```python
from build123d import *

# Parameters (mm, degrees)
SKETCH1_W                                         = 172.72
SKETCH1_H                                         = 64.77
BOSS_EXTRUDE1_DEPTH                               = 1.5875
CSK_FOR_8_FLAT_HEAD_MACHINE_SCREW_100_D           = 4.4958
CSK_FOR_8_FLAT_HEAD_MACHINE_SCREW_100_DEPTH       = 12.7
CSK_FOR_8_FLAT_HEAD_MACHINE_SCREW_100_CSINK_D     = 8.4328
CSK_FOR_8_FLAT_HEAD_MACHINE_SCREW_100_CSINK_ANGLE = 100
CSK_FOR_8_FLAT_HEAD_MACHINE_SCREW_100_TIP         = 1.350674586


with BuildPart() as part:
    # Sketch1 → Boss-Extrude1 (new body)
    with BuildSketch(Plane(origin=(0, 0, 0), x_dir=(1, 0, 0), z_dir=(0, 1, 0))):
        with Locations((86.36, 32.385)):
            Rectangle(SKETCH1_W, SKETCH1_H)
    extrude(amount=BOSS_EXTRUDE1_DEPTH)

    # CSK for #8 Flat Head Machine Screw (100)1
    with Locations(Plane(origin=(0, 1.5875, 0), x_dir=(1, 0, 0), z_dir=(0, 1, 0))):
        with Locations((12.7, 54.61), (38.1, 54.61), (63.5, 54.61), (109.22, 54.61), (134.62, 54.61), (160.02, 54.61), (160.02, 10.16), (134.62, 10.16), (109.22, 10.16), (63.5, 10.16), (38.1, 10.16), (12.7, 10.16)):
            CounterSinkHole(CSK_FOR_8_FLAT_HEAD_MACHINE_SCREW_100_D / 2, CSK_FOR_8_FLAT_HEAD_MACHINE_SCREW_100_CSINK_D / 2, depth=CSK_FOR_8_FLAT_HEAD_MACHINE_SCREW_100_DEPTH, counter_sink_angle=CSK_FOR_8_FLAT_HEAD_MACHINE_SCREW_100_CSINK_ANGLE)
            with Locations((0, 0, -(CSK_FOR_8_FLAT_HEAD_MACHINE_SCREW_100_DEPTH + CSK_FOR_8_FLAT_HEAD_MACHINE_SCREW_100_TIP / 2))):  # 118° drill point
                Cone(0, CSK_FOR_8_FLAT_HEAD_MACHINE_SCREW_100_D / 2, CSK_FOR_8_FLAT_HEAD_MACHINE_SCREW_100_TIP, mode=Mode.SUBTRACT)


solid = part.part
```
Geometry check sheet. Reference: the model listing, model coordinates, mm. Coordinates: 2 decimals unless noted, no trailing zeros. Order: outer loops, then holes, each group sorted by start corner. A loop starts at its lowest first (then second) coordinate and runs counter-clockwise, first axis right, second up.
Q1. Sectioned sample at B-B on y = 1.05. Give the number of separate pieces and of enclosed holes in the cut face, and give its area (3 significant figures).
Reply:
separate pieces: 1
enclosed holes: 12
area: 10,700 mm2
Q2. Sectioned sample at C-C on x = 12.7. Record the cut outline in (y, z), and give its area (3 significant figures).
Reply:
outline: (0, -64.77) - (1.59, -64.77) - (1.59, -58.83) - (0, -56.93) - close; (0, -52.29) - (1.59, -50.39) - (1.59, -14.38) - (0, -12.48) - close; (0, -7.84) - (1.59, -5.94) - (1.59, 0) - (0, 0) - close
area: 82.1 mm2
Q3. Sectioned sample at A-A on z = -10.16. Record the cut outline in (x, y).
Reply:
outline: (0, 0) - (10.38, 0) - (8.48, 1.59) - (0, 1.59) - close; (15.02, 0) - (35.78, 0) - (33.88, 1.59) - (16.92, 1.59) - close; (40.42, 0) - (61.18, 0) - (59.28, 1.59) - (42.32, 1.59) - close; (65.82, 0) - (106.9, 0) - (105, 1.59) - (67.72, 1.59) - close; (111.54, 0) - (132.3, 0) - (130.4, 1.59) - (113.44, 1.59) - close; (136.94, 0) - (157.7, 0) - (155.8, 1.59) - (138.84, 1.59) - close; (162.34, 0) - (172.72, 0) - (172.72, 1.59) - (164.24, 1.59) - close
Q4. Thickness scan on probe 1 along Z at (x, y) = (13, 0.7); probe 2 along Z at (x, y) = (39.5, 0.55); probe 3 along Y at (x, z) = (138, -53.5). Record the ranges inside material, lowest first.
Reply:
probe 1: z = -64.77 to -57.75, -51.47 to -13.3, -7.02 to 0
probe 2: z = -64.77 to -57.24, -51.98 to -12.79, -7.53 to 0
probe 3: y = 0 to 1.03
